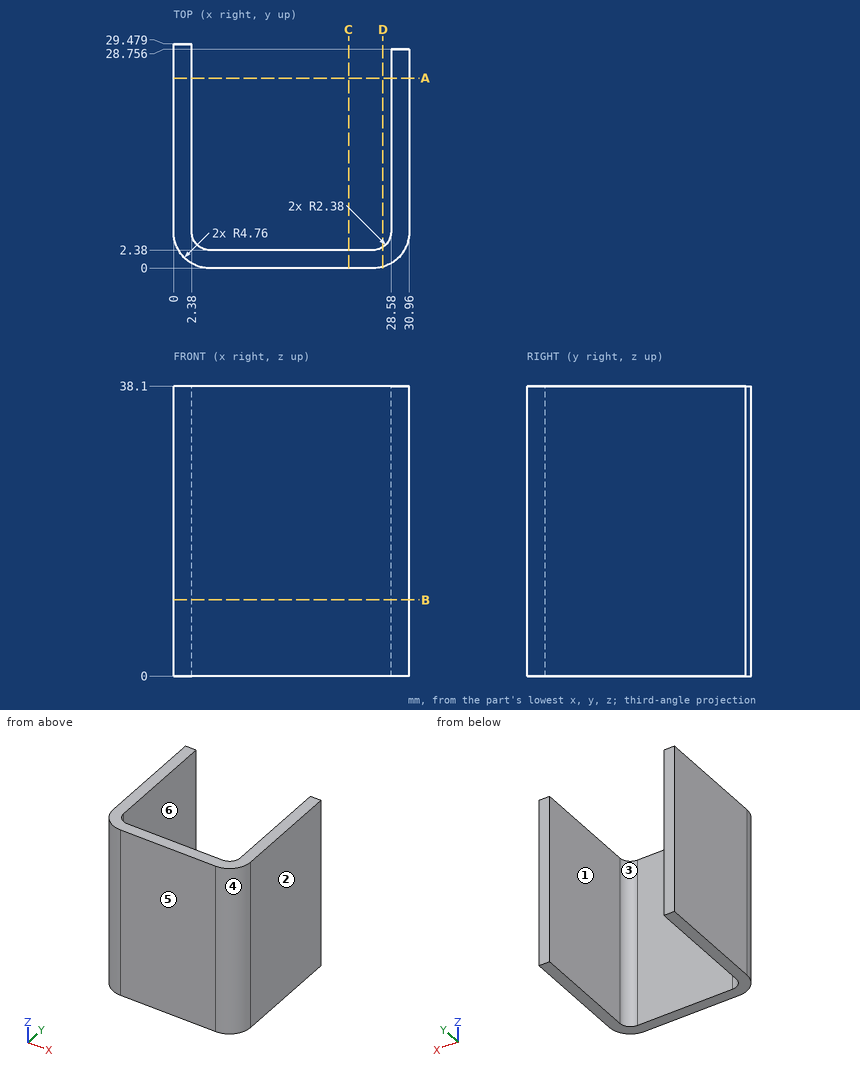
Can you work these out from the drawing? Everything is in mm from the part's minimum corner. A direction names the side the tool comes from. Give positions to 0.01 mm unless a question says otherwise; leave off trailing zeros. Order: outer loops, then holes, each group sorted by start corner. A loop starts at its lowest first (then second) coordinate and runs counter-clockwise, first axis right, second up. Notation, with made-up numbers: (67, -1) -> (124, -1) arc R21 ccw to (124, 31) -> close; hole circle Ø9 at (28.5, 84). An arc over 180 degrees is marked (long way). Return JSON: item names as keys, results as strings.
1. Imagine slicing it at B-B on z = 10. List the corners of the cut face in (x, y) for me (1 decimal).
Answer list:
{"outline": "(0, 4.8) arc R4.8 ccw to (4.8, 0) -> (26.2, 0) arc R4.8 ccw to (31, 4.8) -> (31, 28.8) -> (28.6, 28.8) -> (28.6, 4.8) arc R2.4 cw to (26.2, 2.4) -> (4.8, 2.4) arc R2.4 cw to (2.4, 4.8) -> (2.4, 29.5) -> (0, 29.5) -> close"}
2. I need wall thicknesses on line 1 (X direction, y = 17, z = 13); line 2 (Y direction, x = 18, z = 3); line 3 (Y direction, x = 3, z = 3) (1 decimal). Which ranges of each line are inside material? Lowest first, please. Write a range as from..to.
Answer list:
{"line 1": "x = 0..2.38, 28.58..30.96", "line 2": "y = 0..2.38", "line 3": "y = 0.3..3.2"}
3. Imagine slicing it at A-A on y = 25. List the corners of the cut face in (x, z) for me.
Answer list:
{"outline": "(0, 0) -> (2.38, 0) -> (2.38, 38.1) -> (0, 38.1) -> close; (28.58, 0) -> (30.96, 0) -> (30.96, 38.1) -> (28.58, 38.1) -> close"}
4. Thinking about a two-plate mould opening in X: for the marked faces 3, 4, 5 and 6, which applies, pulls with the +X half, pulls with the -X half, needs draft (parallel to the pull), parting line crosses it, or undercut?
Answer list:
{"face 3": "undercut", "face 4": "pulls with the +X half", "face 5": "needs draft", "face 6": "undercut"}
5. Imagine slicing it at C-C on x = 23. List the corners of the cut face in (y, z) for me.
Answer list:
{"outline": "(0, 0) -> (2.38, 0) -> (2.38, 38.1) -> (0, 38.1) -> close"}
6. On a 3-axis mill with a long thin cutter (end or side, diameter ignored), from which of +Z, -Z, +X, -X, +Y, -Y can I reach the whole of each face in a straight line? I mean the marked faces 1 and 2. Say none if no direction works.
Answer list:
{"face 1": "+Z, -Z, +Y", "face 2": "+Z, -Z, +X, +Y, -Y"}
7. For pin 1 Ø5 at (y, z) = (13, 20.5) entering from -X; pin 2 Ø12 at (x, z) = (11, 5) entering from +Y; pin 3 Ø3 at (x, y) = (4.5, 4.5) entering from +Z; pin 4 Ø17 at (x, z) = (11.5, 23) entering from +Y, each with a flat end and sliding along its axis, tell me the tip position at first contact or that it passes through.
Answer list:
{"pin 1": "stops at x = 0", "pin 2": "stops at y = 2.38", "pin 3": "passes through", "pin 4": "stops at y = 3.16"}
8. Imagine slicing it at D-D on x = 27.5. List the corners of the cut face in (y, z) for me.
Answer list:
{"outline": "(0.18, 0) -> (2.77, 0) -> (2.77, 38.1) -> (0.18, 38.1) -> close"}
